Job drawing, mm, ordinate dimensions from the low corner. One solid piece. Round coordinates to 2 decimals unless told otherwise and drop trailing zeros. Loops run counter-clockwise (first coordinate to the right, second up) from the corner with the lowest first, then second, coordinate; pieces in that order, holes last.
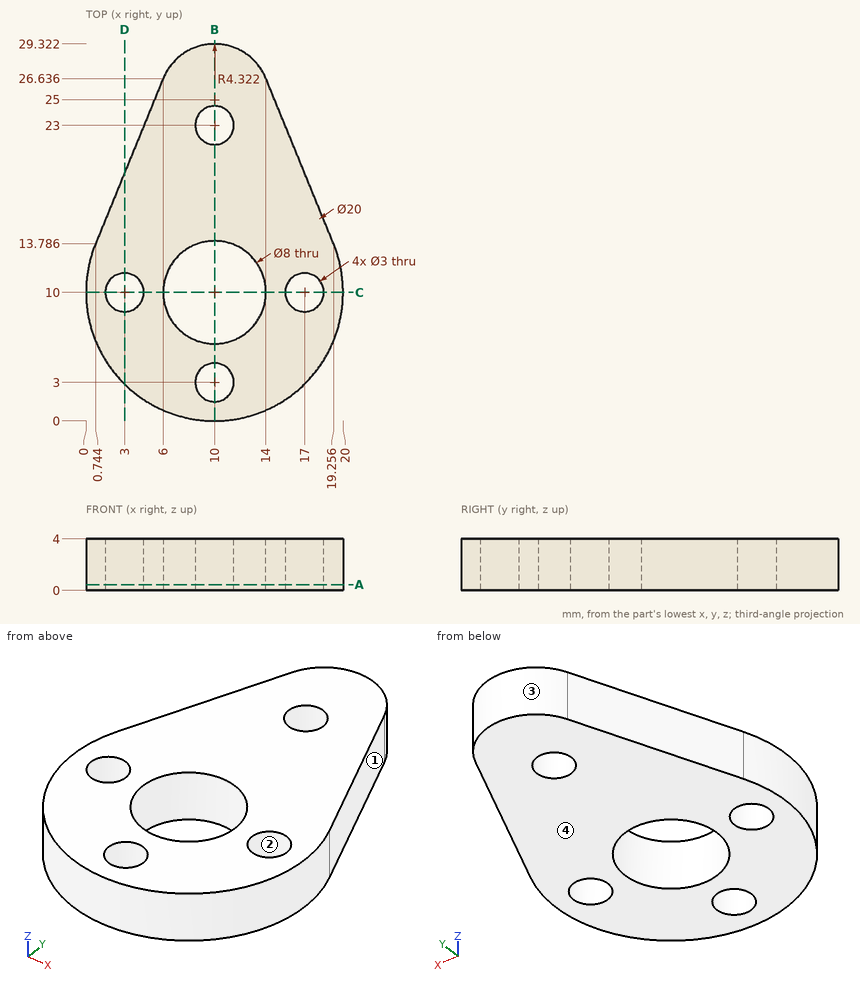
Item 1: Cut at C-C, the plane y = 10. Give the cut face in (x, z), plus the area to 3 significant figures.
Answers follow:
outline: (0, 0) - (1.5, 0) - (1.5, 4) - (0, 4) - close; (4.5, 0) - (6, 0) - (6, 4) - (4.5, 4) - close; (14, 0) - (15.5, 0) - (15.5, 4) - (14, 4) - close; (18.5, 0) - (20, 0) - (20, 4) - (18.5, 4) - close
area: 24.0 mm2
Item 2: Cut at B-B, the plane x = 10. Give the cut face in (y, z).
Answers follow:
outline: (0, 0) - (1.5, 0) - (1.5, 4) - (0, 4) - close; (4.5, 0) - (6, 0) - (6, 4) - (4.5, 4) - close; (14, 0) - (21.5, 0) - (21.5, 4) - (14, 4) - close; (24.5, 0) - (29.32, 0) - (29.32, 4) - (24.5, 4) - close
Item 3: Flat gauge pins, fed straight in: P1, Ø1, axis at x = 11.5, z = 0.5, coming from the +Y side (1 decimal); P2, Ø1, axis at y = 6.5, z = 1, coming from the +X side. Where does each tip first touch, or does it go through?
Answers follow:
P1: stops at y = 29.2
P2: stops at x = 19.54
Item 4: Cut at A-A, the plane z = 0.45. Give the cut face in (x, y) (1 decimal).
Answers follow:
outline: (0.7, 13.8) arc R10 ccw (long way) to (19.3, 13.8) - (14, 26.6) arc R4.3 ccw to (6, 26.6) - close; hole circle Ø3 at (3, 10); hole circle Ø8 at (10, 10); hole circle Ø3 at (10, 3); hole circle Ø3 at (10, 23); hole circle Ø3 at (17, 10)
Item 5: Two-plate mould, pull along X, no slides. Class the marked faces 1, 2, 3 and 4: released by +X, released by -X, zero draft, split by the parting line, or undercut.
Answers follow:
face 1: released by +X
face 2: undercut
face 3: split by the parting line
face 4: zero draft
Item 6: Cut at D-D, the plane x = 3. Give the cut face in (y, z).
Answers follow:
outline: (2.86, 0) - (8.5, 0) - (8.5, 4) - (2.86, 4) - close; (11.5, 0) - (19.3, 0) - (19.3, 4) - (11.5, 4) - close
Item 7: Probe line 1 (Y direction, x = 10, z = 2.85); line 2 (Y direction, x = 13.5, z = 3.8) (1 decimal); line 3 (Y direction, x = 3, z = 2.3) (1 decimal). List the from-to ranges inside material, lowest first.
Answers follow:
line 1: y = 0 to 1.5, 4.5 to 6, 14 to 21.5, 24.5 to 29.32
line 2: y = 0.6 to 8.1, 11.9 to 27.5
line 3: y = 2.9 to 8.5, 11.5 to 19.3
